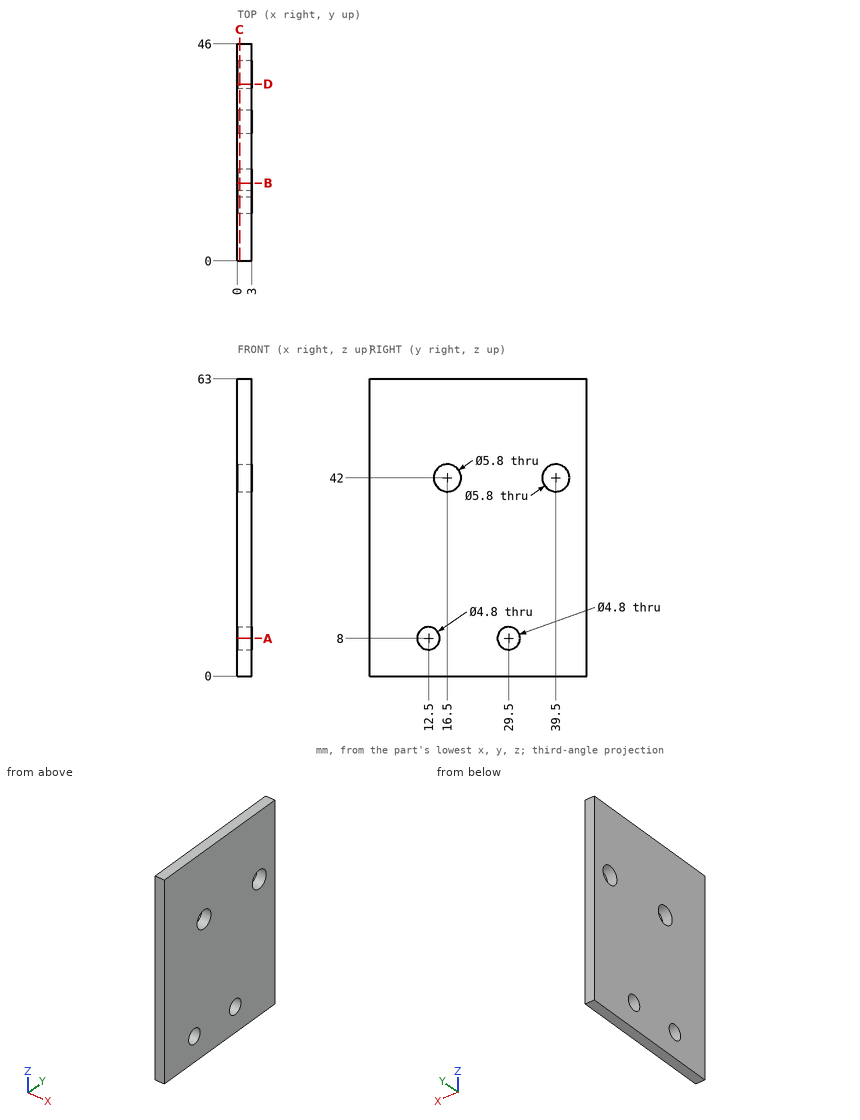
Source: three-view drawing plus pictorial views. Frame: mm from the lowest corner of the part. Coordinates: 2 decimals unless noted, no trailing zeros. Write each loop counter-clockwise with the first axis right and the second up, starting at its lowest first coordinate (ties: lowest second). Pieces come first, ordered by that corner, then holes. Notation, with made-up numbers: (14.5, -27) -> (54.5, -27) arc R14 cw to (54.5, -1) -> close; hole circle Ø9 at (68.5, -34.5). An arc over 180 degrees is marked (long way). Write each question's results on one line, items separated by ' | '.
Item 1: Section query B-B on y = 16.5. Return loops of the section in (x, z), plus the area to 3 significant figures.
Conclusion:
outline: (0, 0) -> (3, 0) -> (3, 39.1) -> (0, 39.1) -> close; (0, 44.9) -> (3, 44.9) -> (3, 63) -> (0, 63) -> close | area: 172 mm^2
Item 2: Material intervals for probe 1 along Z at (x, y) = (2.15, 29.5); probe 2 along Z at (x, y) = (2.25, 15.5), sorted ascending.
Conclusion:
probe 1: z = 0 to 5.6, 10.4 to 63 | probe 2: z = 0 to 39.28, 44.72 to 63
Item 3: Pin query (flat end, axial travel): pin 1 Ø3 at (y, z) = (12.5, 8) entering from +X. Return the tip coordinate at first contact, or that it passes through.
Conclusion:
pin 1: passes through
Item 4: Section query D-D on y = 37.5. Return loops of the section in (x, z).
Conclusion:
outline: (0, 0) -> (3, 0) -> (3, 39.9) -> (0, 39.9) -> close; (0, 44.1) -> (3, 44.1) -> (3, 63) -> (0, 63) -> close
Item 5: Section query C-C on x = 0.45. Return loops of the section in (y, z), plus the area to 3 significant figures.
Conclusion:
outline: (0, 0) -> (46, 0) -> (46, 63) -> (0, 63) -> close; hole circle Ø4.8 at (12.5, 8); hole circle Ø5.8 at (16.5, 42); hole circle Ø4.8 at (29.5, 8); hole circle Ø5.8 at (39.5, 42) | area: 2,810 mm^2
Item 6: Section query A-A on z = 8. Return loops of the section in (x, y).
Conclusion:
outline: (0, 0) -> (3, 0) -> (3, 10.1) -> (0, 10.1) -> close; (0, 14.9) -> (3, 14.9) -> (3, 27.1) -> (0, 27.1) -> close; (0, 31.9) -> (3, 31.9) -> (3, 46) -> (0, 46) -> close
